Work out the finished part from the listing and answer in its coordinate system (mm). Face numbers are marked on the shaded views. Coordinates: 2 decimals unless noted, no trailing zeros. Write each loop counter-clockwise with the first axis right and the second up, starting at its lowest first coordinate (ties: lowest second). Pieces come first, ordered by that corner, then holes. Notation, with made-up numbers: M -12.5,-28.75 L 41.5,-28.75 A27 cw 41.5,10.25 Z; hole C -38.5,70 d4. An arc over 180 degrees is marked long. Use CSV: the item, a comma, the result in double quotes.
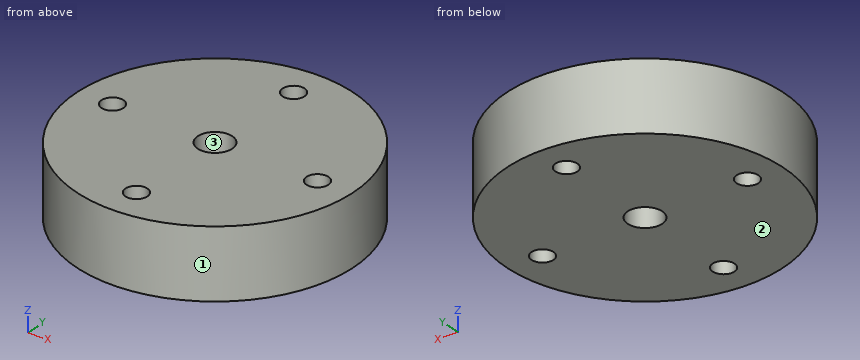
from build123d import *

# Parameters (mm, degrees)
SKETCH3_R                    = 20
SKETCH3_R_2                  = 2.5
BOSS_EXTRUDE2_DEPTH          = 10
F_1_8_0_125_DIAMETER_HOLE2_D = 3.175


with BuildPart() as part:
    # Sketch3 → Boss-Extrude2 (new body)
    with BuildSketch(Plane.XY):
        Circle(SKETCH3_R)
        Circle(SKETCH3_R_2, mode=Mode.SUBTRACT)
    extrude(amount=BOSS_EXTRUDE2_DEPTH)

    # 1/8 (0.125) Diameter Hole2 (through all)
    with Locations(Plane.XY.offset(10)):
        with Locations((0, 15), (15, 0), (0, -15), (-15, 0)):
            Hole(F_1_8_0_125_DIAMETER_HOLE2_D / 2)


solid = part.part
Item 1: The part is cut by section A-A (x = 0.5). Write down the section's boundary in (y, z), then the cut area to 3 significant figures.
Answer:
outline,"M -19.99,0 L -16.51,0 L -16.51,10 L -19.99,10 Z; M -13.49,0 L -2.45,0 L -2.45,10 L -13.49,10 Z; M 2.45,0 L 13.49,0 L 13.49,10 L 2.45,10 Z; M 16.51,0 L 19.99,0 L 19.99,10 L 16.51,10 Z"
area,"291 mm2"
Item 2: The part is cut by section B-B (z = 1). Write down the section's boundary in (x, y) (1 decimal).
Answer:
outline,"C 0,0 d40; hole C -15,0 d3.2; hole C 0,0 d5; hole C 0,-15 d3.2; hole C 0,15 d3.2; hole C 15,0 d3.2"
Item 3: Given pin 1 (6.5 mm diameter, centred on x = 0, y = 0, fed in from +Z); pin 2 (1.9 mm diameter, centred on x = -15, y = 0, fed in from -Z); pin 3 (1.5 mm diameter, centred on x = -2, z = 9, fed in from +Y); pin 4 (4 mm diameter, centred on x = -5.5, z = 3, fed in from +Y), each flat-ended and moving along its own axis, determine where each tip first touches the part or whether it passes through.
Answer:
pin 1,"stops at z = 10"
pin 2,"passes through"
pin 3,"stops at y = 19.96"
pin 4,"stops at y = 19.69"
Item 4: For a pull along X with two mould halves and no side action, classify the marked faces 1, 2 and 3 as released by +X, released by -X, zero draft, split by the parting line, or undercut.
Answer:
face 1,"split by the parting line"
face 2,"zero draft"
face 3,"undercut"
Item 5: Consider probe 1 along Y at (x, z) = (0, 4.5); probe 2 along Y at (x, z) = (-1, 6.5); probe 3 along Y at (x, z) = (-15, 5). Determine where each line is inside the solid, lowest interval first.
Answer:
probe 1,"y = -20 to -16.59, -13.41 to -2.5, 2.5 to 13.41, 16.59 to 20"
probe 2,"y = -19.97 to -16.23, -13.77 to -2.29, 2.29 to 13.77, 16.23 to 19.97"
probe 3,"y = -13.23 to -1.59, 1.59 to 13.23"
Item 6: The part is cut by section C-C (y = -15.5). Write down the section's boundary in (x, z), then the cut area to 3 significant figures.
Answer:
outline,"M -12.64,0 L -1.51,0 L -1.51,10 L -12.64,10 Z; M 1.51,0 L 12.64,0 L 12.64,10 L 1.51,10 Z"
area,"223 mm2"
